Could you check a few things on this drawing? It's one solid part, dimensions in mm from its lowest x, y, z. A direction names the side the tool comes from. Give positions to 0.01 mm unless a question says otherwise; leave off trailing zeros. Write each loop counter-clockwise with the first axis right and the second up, starting at its lowest first coordinate (ties: lowest second). Pieces come first, ordered by that corner, then holes. Notation, with made-up numbers: M -21,51.25 L -3,51.25 A10 ccw -3,66.25 Z; hole C 4.5,13.5 d7. An arc over 180 degrees is marked long. Write each question's results on one line, items separated by ' | '. Start each with the question number.
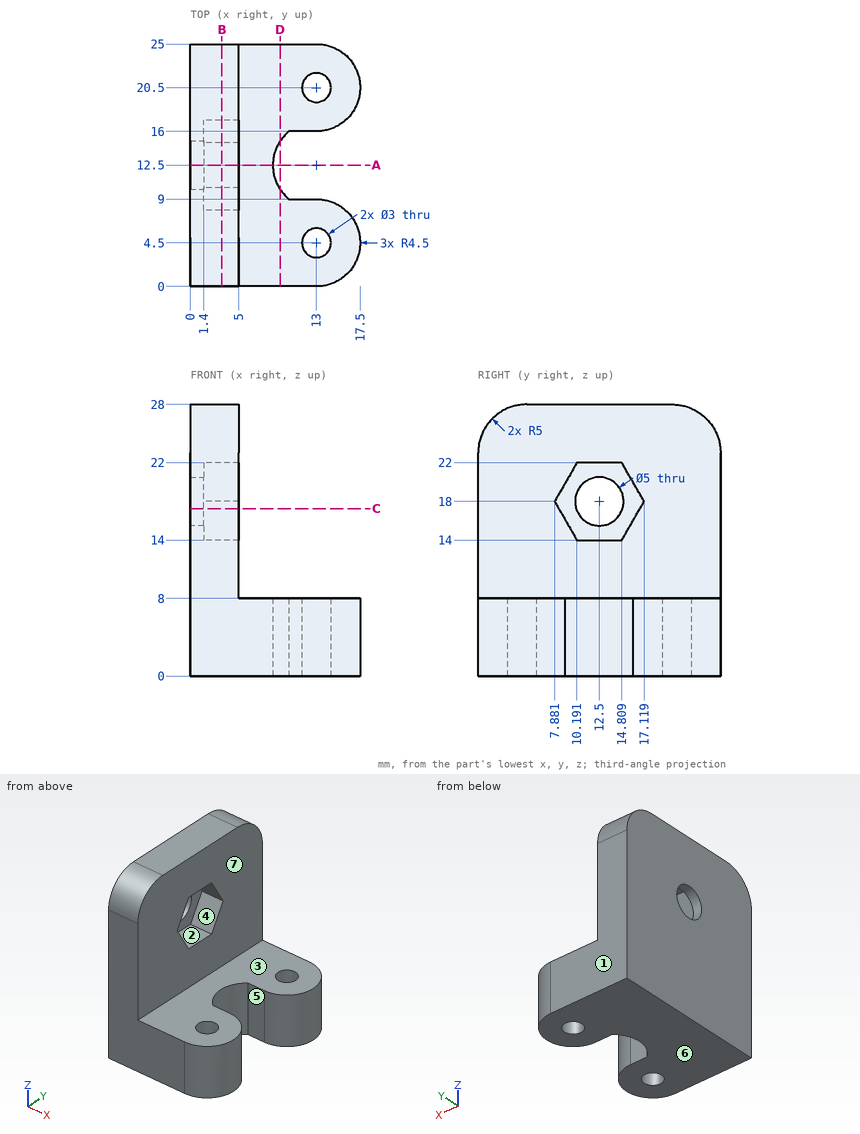
Q1. For the marked faces 5, 6 and 7, which set-ups out of +Z, -Z, +X, -X, +Y, -Y let a thin tool reach every point of the face, with its end or its side?
Q2. I'm going to push flat-ended pins straight in: P1, Ø6.5, axis at y = 11, z = 16, coming from the +X side; P2, Ø4, axis at x = 15.5, z = 6, coming from the -Y side; P3, Ø4, axis at x = 13, y = 4.5, coming from the +Z side. Where does each tip first touch, or does it pass through?
Q3. If we section it at B-B (x = 3.25): Please give me the cut outline in (y, z).
Q4. If we section it at A-A (y = 12.5): Please give me the cut outline in (x, z).
Q5. If we section it at D-D (x = 9.25): Please give me the cut outline in (y, z), plus the area to 3 significant figures.
Q6. If we section it at C-C (z = 17.25): Please give me the cut outline in (x, y) (1 decimal).
Q7. Please list where these lines run through material, in increasing order: line 1 (Z direction, x = 2.25, y = 12.75); line 2 (X direction, y = 23, z = 19.75); line 3 (Z direction, x = 5.25, y = 22.25). Write a range as [from, to].
Q8. If we mould it in two halves opening along Z, with no side actions, what happens to the marked faces 1, 2, 3 and 4? For each: pulls with the +Z half, pulls with the -Z half, needs draft (parallel to the pull), parting line crosses it, or undercut.
Determined:
1) face 5: +Z, -Z, +X | face 6: -Z, +X, -X, +Y, -Y | face 7: +Z, +X, +Y, -Y
2) P1: stops at x = 5 | P2: stops at y = 0.03 | P3: stops at z = 8
3) outline: M 0,0 L 25,0 L 25,23 A5 ccw 20,28 L 5,28 A5 ccw 0,23 Z; hole M 7.88,18 L 10.19,14 L 14.81,14 L 17.12,18 L 14.81,22 L 10.19,22 Z
4) outline: M 0,0 L 8.5,0 L 8.5,8 L 5,8 L 5,14 L 1.4,14 L 1.4,15.5 L 0,15.5 Z; M 0,20.5 L 1.4,20.5 L 1.4,22 L 5,22 L 5,28 L 0,28 Z
5) outline: M 0,0 L 10.01,0 L 10.01,8 L 0,8 Z; M 14.99,0 L 25,0 L 25,8 L 14.99,8 Z | area: 160 mm²
6) outline: M 0,0 L 5,0 L 5,8.3 L 1.4,8.3 L 1.4,10.1 L 0,10.1 Z; M 0,14.9 L 1.4,14.9 L 1.4,16.7 L 5,16.7 L 5,25 L 0,25 Z
7) line 1: z = [0, 14], [22, 28] | line 2: x = [0, 5] | line 3: z = [0, 8]
8) face 1: needs draft | face 2: undercut | face 3: pulls with the +Z half | face 4: undercut
